from build123d import *

# Parameters (mm, degrees)
SKETCH_1_R      = 1.35
SKETCH_1_W      = 29.2
SKETCH_1_H      = 55.7
EXTRUDE_1_DEPTH = 2
FILLET_1_R      = 2


with BuildPart() as part:
    # 草图1 → 凸台-拉伸1 (new body)
    with BuildSketch(Plane(origin=(0, 0, 0), x_dir=(1, 0, 0), z_dir=(0, 1, 0))):
        Polygon((-35, -33.35), (-35, -41.85), (35, -41.85), (35, -33.35), (75, -33.35), (75, 33.35), (35, 33.35), (35, 52.35), (-35, 52.35), (-35, 33.35), (-75, 33.35), (-75, -33.35), align=None)
        with Locations(Location((-72.2, 18.75, 0), (0, 0, 270))):
            Circle(SKETCH_1_R, mode=Mode.SUBTRACT)
        with Locations(Location((-72.2, -3.25, 0), (0, 0, 270))):
            Circle(SKETCH_1_R, mode=Mode.SUBTRACT)
        with Locations(Location((-72.2, -25.25, 0), (0, 0, 270))):
            Circle(SKETCH_1_R, mode=Mode.SUBTRACT)
        with Locations(Location((-37.6, -25.25, 0), (0, 0, 90))):
            Circle(SKETCH_1_R, mode=Mode.SUBTRACT)
        with Locations(Location((-37.6, -3.25, 0), (0, 0, 90))):
            Circle(SKETCH_1_R, mode=Mode.SUBTRACT)
        with Locations(Location((-37.6, 18.75, 0), (0, 0, 90))):
            Circle(SKETCH_1_R, mode=Mode.SUBTRACT)
        with Locations(Location((37.6, 18.75, 0), (0, 0, 270))):
            Circle(SKETCH_1_R, mode=Mode.SUBTRACT)
        with Locations(Location((37.6, -3.25, 0), (0, 0, 270))):
            Circle(SKETCH_1_R, mode=Mode.SUBTRACT)
        with Locations(Location((37.6, -25.25, 0), (0, 0, 270))):
            Circle(SKETCH_1_R, mode=Mode.SUBTRACT)
        with Locations(Location((72.2, -25.25, 0), (0, 0, 90))):
            Circle(SKETCH_1_R, mode=Mode.SUBTRACT)
        with Locations(Location((72.2, -3.25, 0), (0, 0, 90))):
            Circle(SKETCH_1_R, mode=Mode.SUBTRACT)
        with Locations(Location((72.2, 18.75, 0), (0, 0, 90))):
            Circle(SKETCH_1_R, mode=Mode.SUBTRACT)
        with Locations(Location((-43.9, -30.55, 0), (0, 0, 270))):
            Circle(SKETCH_1_R, mode=Mode.SUBTRACT)
        with Locations(Location((-65.9, -30.55, 0), (0, 0, 90))):
            Circle(SKETCH_1_R, mode=Mode.SUBTRACT)
        with Locations(Location((43.9, -30.55, 0), (0, 0, 90))):
            Circle(SKETCH_1_R, mode=Mode.SUBTRACT)
        with Locations(Location((65.9, -30.55, 0), (0, 0, 270))):
            Circle(SKETCH_1_R, mode=Mode.SUBTRACT)
        with Locations((-54.9, 0)):
            Rectangle(SKETCH_1_W, SKETCH_1_H, mode=Mode.SUBTRACT)
        with Locations((54.9, 0)):
            Rectangle(SKETCH_1_W, SKETCH_1_H, mode=Mode.SUBTRACT)
        with BuildLine():
            Line((-15, 49.85), (15, 49.85))
            ThreePointArc((15, 49.85), (16, 48.85), (15, 47.85))
            Line((15, 47.85), (-15, 47.85))
            ThreePointArc((-15, 47.85), (-16, 48.85), (-15, 49.85))
        make_face(mode=Mode.SUBTRACT)
    extrude(amount=EXTRUDE_1_DEPTH)

    # 圆角1
    fillet_1_edges = [part.edges().sort_by_distance(p)[0] for p in [
        (-35, 1, -52.35),
        (35, 1, -52.35),
        (35, 1, -33.35),
        (35, 1, 33.35),
        (35, 1, 41.85),
        (-35, 1, 41.85),
        (-35, 1, 33.35),
        (-75, 1, 33.35),
        (-75, 1, -33.35),
        (-35, 1, -33.35),
        (-40.3, 1, 27.85),
        (-40.3, 1, -27.85),
        (-69.5, 1, -27.85),
        (-69.5, 1, 27.85),
        (69.5, 1, 27.85),
        (69.5, 1, -27.85),
        (40.3, 1, -27.85),
        (40.3, 1, 27.85),
    ]]
    fillet(fillet_1_edges, radius=FILLET_1_R)


solid = part.part
The listing builds one solid part. Answer for the finished solid, in the listing's coordinates (mm). Give positions to 0.01 mm unless a question says otherwise; leave off trailing zeros. Write each loop counter-clockwise with the first axis right and the second up, starting at its lowest first coordinate (ties: lowest second). Pieces come first, ordered by that corner, then holes. Notation, with made-up numbers: (31.25, -31) - (40.25, -31) arc R15 cw to (40.25, -22) - close; hole circle Ø7 at (80.5, 35.5). An arc over 180 degrees is marked (long way). Use a Markdown table: item, result.
1. Each of these flat-tipped pins is pushed along its axis until it touches: P1, Ø0.6, axis at x = -58, y = 1.5, coming from the -Z side; P2, Ø1.6, axis at x = -72.2, z = 25.25, coming from the +Y side; P3, Ø0.6, axis at y = 1, z = 38, coming from the +X side. Where does it stop, or does it pass through?
Values follow:
| item | result |
|---|---|
| P1 | stops at z = -33.35 |
| P2 | passes through |
| P3 | stops at x = 35 |
2. Find the intervals of material crossed by probe 1 along X at (y, z) = (1.4, -17); probe 2 along Z at (x, y) = (72.2, 1.5); probe 3 along X at (y, z) = (0.95, 30.55), in increasing order. Write a range as from..to.
Values follow:
| item | result |
|---|---|
| probe 1 | x = -75..-69.5, -40.3..40.3, 69.5..75 |
| probe 2 | z = -33.35..-20.1, -17.4..1.9, 4.6..23.9, 26.6..33.35 |
| probe 3 | x = -75..-67.25, -64.55..-45.25, -42.55..42.55, 45.25..64.55, 67.25..75 |
3. Section D-D on x = -7 is taken. Write down the section's boundary in (y, z), plus the area to 3 significant figures.
Values follow:
| item | result |
|---|---|
| outline | (0, -52.35) - (2, -52.35) - (2, -49.85) - (0, -49.85) - close; (0, -47.85) - (2, -47.85) - (2, 41.85) - (0, 41.85) - close |
| area | 184 mm² |
4. For a pull along X with two mould halves and no side action, classify faces 1 (the flat face through (-1, 2, -6)), 2 (the cylindrical face through (-38.006, 0.986, -20.038)) as released by +X, released by -X, zero draft, split by the parting line, or undercut.
Values follow:
| item | result |
|---|---|
| face 1 | zero draft |
| face 2 | undercut |
5. Section C-C on y = 1.1 is taken. Count the separate pieces of the cut face and the enclosed holes in it, plus the area to 3 significant figures.
Values follow:
| item | result |
|---|---|
| separate pieces | 1 |
| enclosed holes | 19 |
| area | 8,530 mm² |
6. Section B-B on x = 48 is taken. Write down the section's boundary in (y, z).
Values follow:
| item | result |
|---|---|
| outline | (0, -33.35) - (2, -33.35) - (2, -27.85) - (0, -27.85) - close; (0, 27.85) - (2, 27.85) - (2, 33.35) - (0, 33.35) - close |
7. Section A-A on z = -9 is taken. Write down the section's boundary in (x, y).
Values follow:
| item | result |
|---|---|
| outline | (-75, 0) - (-69.5, 0) - (-69.5, 2) - (-75, 2) - close; (-40.3, 0) - (40.3, 0) - (40.3, 2) - (-40.3, 2) - close; (69.5, 0) - (75, 0) - (75, 2) - (69.5, 2) - close |
